```python
from build123d import *

# Parameters (mm, degrees)
SKETCH_1_R          = 3.8
EXTRUDE_1_DEPTH     = 4
SKETCH_2_W          = 9.2
SKETCH_2_H          = 9.2
EXTRUDE_2_DEPTH     = 0.5
FILLET_1_R          = 0.4
SKETCH_7_RX         = 2
SKETCH_7_RY         = 0.5
SKETCH_7_R          = 0.8
CUT_EXTRUDE_4_DEPTH = 4
SKETCH_8_R          = 0.6
CUT_EXTRUDE_5_DEPTH = 8.636753237


with BuildPart() as part:
    # Эскиз1 → Бобышка-Вытянуть1 (new body)
    with BuildSketch(Plane.XY):
        Circle(SKETCH_1_R)
    extrude(amount=EXTRUDE_1_DEPTH)

    # Эскиз2 → Бобышка-Вытянуть2 (add)
    with BuildSketch(Plane(origin=(0, 0, 0), x_dir=(-1, 0, 0), z_dir=(0, 0, -1))):
        Rectangle(SKETCH_2_W, SKETCH_2_H)
    extrude(amount=EXTRUDE_2_DEPTH)

    # Скругление1
    fillet_1_edges = [part.edges().sort_by_distance(p)[0] for p in [
        (-3.8, 0, 4),
    ]]
    fillet(fillet_1_edges, radius=FILLET_1_R)

    # Эскиз7 → Вырез-Вытянуть4 (cut)
    with BuildSketch(Plane.XY.offset(4)):
        with BuildLine():
            ThreePointArc((0.780530418, 1.824579743), (0, 1.2), (-0.780530418, 1.824579743))
            ThreePointArc((-0.780530418, 1.824579743), (-1.785343213, 0.036245206), (-2, -2.003782154))
            add(Edge.make_bspline(
                [(2, -2.003782154), (2, -1.503782154), (0, -1.503782154), (-2, -1.503782154), (-2, -2.003782154)],
                knots=[0, 0, 0, 1.570796327, 1.570796327, 3.141592654, 3.141592654, 3.141592654], degree=2, weights=[1, 0.707106781, 1, 0.707106781, 1]))
            ThreePointArc((2, -2.003782154), (1.785343213, 0.036245206), (0.780530418, 1.824579743))
        make_face()
        with Locations((0, -2.003782154)):
            Ellipse(SKETCH_7_RX, SKETCH_7_RY)
        with Locations((0, 2)):
            Circle(SKETCH_7_R)
    extrude(amount=-CUT_EXTRUDE_4_DEPTH, mode=Mode.SUBTRACT)

    # Эскиз8 → Вырез-Вытянуть5 (cut, through all)
    with BuildSketch(Plane.XY):
        Circle(SKETCH_8_R)
    extrude(amount=-CUT_EXTRUDE_5_DEPTH, mode=Mode.SUBTRACT)


solid = part.part
```
Build history of the part. All positions in model axes, mm. A direction names the side the tool comes from. Give positions to 0.01 mm unless a question says otherwise; leave off trailing zeros. Loops run counter-clockwise (first coordinate to the right, second up) from the corner with the lowest first, then second, coordinate; pieces in that order, holes last. Notation, with made-up numbers: (-27, 73.5) -> (32, 73.5) arc R14 ccw to (32, 87.5) -> close; hole circle Ø7 at (65.25, 24.25). An arc over 180 degrees is marked (long way). One line per question, with ' | ' between items. Start each with the question number.
1) 3-axis set-ups, long thin cutter, end or side, ignore diameter. For faces 1 (the flat face through (0, -1, 0)), 2 (the cylindrical face through (0.323, 0.506, -0.246)): which of +Z, -Z, +X, -X, +Y, -Y reach the whole face in a straight line?
2) Probe L1, parallel to Y at x = 0, z = -0.4; L2, parallel to Z at x = -0.75, y = -0.75; L3, parallel to X at y = -0.5, z = 2.1. List the from-to ranges inside material, lowest first.
3) Cut at A-A (y = 0). Give the cut face in (x, z), plus the area to 3 significant figures.
4) Two-plate mould, pull along X, no slides. Class faces 3 (the cylindrical face through (-3.796, 0.167, 1.775)), 4 (the flat face through (-2, 1, 4)), 5 (the cylindrical face through (0, 2.8, 2)): released by +X, released by -X, zero draft, split by the parting line, or undercut.
5) Pin check, flat tips, straight feed: pin 1 (4.5 mm diameter, centred on x = 0.5, y = -1, fed in from +Z); pin 2 (1.5 mm diameter, centred on y = 2.5, z = 3, fed in from -X); pin 3 (1 mm diameter, centred on y = -1, z = 2, fed in from -X). Stop position of each tip, or through.
Return value:
1) face 1: +Z | face 2: +Z, -Z
2) L1: -4.6 to -0.6, 0.6 to 4.6 | L2: -0.5 to 0 | L3: -3.77 to -1.92, 1.92 to 3.77
3) outline: (-4.6, -0.5) -> (-0.6, -0.5) -> (-0.6, 0) -> (-1.8, 0) -> (-1.8, 4) -> (-3.4, 4) arc R0.4 ccw to (-3.8, 3.6) -> (-3.8, 0) -> (-4.6, 0) -> close; (0.6, -0.5) -> (4.6, -0.5) -> (4.6, 0) -> (3.8, 0) -> (3.8, 3.6) arc R0.4 ccw to (3.4, 4) -> (1.8, 4) -> (1.8, 0) -> (0.6, 0) -> close | area: 20.0 mm^2
4) face 3: split by the parting line | face 4: zero draft | face 5: undercut
5) pin 1: z = 4 | pin 2: x = -3.37 | pin 3: x = -3.77
